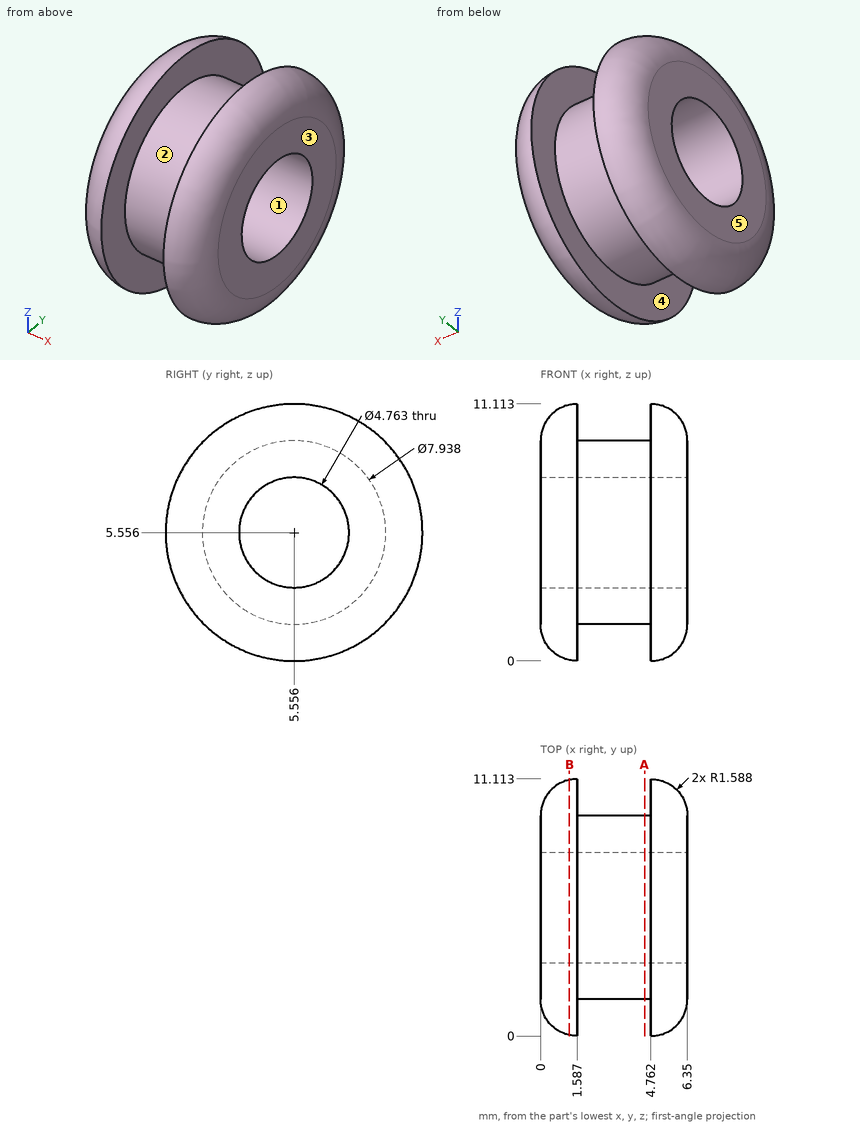
For this review, use the dimensioned drawing (mm, ordinates from the lowest corner) and the shaded views. A direction names the side the tool comes from. Give positions to 0.01 mm unless a question says otherwise; leave off trailing zeros. Order: outer loops, then holes, each group sorted by start corner. A loop starts at its lowest first (then second) coordinate and runs counter-clockwise, first axis right, second up. Notation, with made-up numbers: M 17.25,-3.5 L 60.25,-3.5 A27 ccw 60.25,32.5 Z; hole C -24.75,81 d1. An arc over 180 degrees is marked long. One line per question, with ' | ' between items. Start each with the question number.
1) Wall thickness on L1, parallel to Y at x = 3, z = 6 (1 decimal); L2, parallel to Z at x = 3.75, y = 6.75 (1 decimal): over which ranges is each line inside the solid? List them lowest first. Write a range as from..to.
2) Consider section B-B, the plane x = 1.25. Give the boundary of the cut face in (y, z).
3) For the marked faces 1 and 2, list the 3-axis set-ups (+Z, -Z, +X, -X, +Y, -Y) from which the entire face can be reached by the end or side of a thin tool; tool diameter is ignored.
4) Mouldability with a two-part tool opening along X and no side actions: class the marked faces 3, 4 and 5 as pulls with the +X half, pulls with the -X half, needs draft (parallel to the pull), parting line crosses it, or undercut.
5) Consider section A-A, the plane x = 4.5. Give the boundary of the cut face in (y, z) (1 decimal).
6) Clearance check with flat-ended pins moving along their axes: P1, Ø1.5, axis at x = 2.5, z = 2.5, coming from the +Y side (1 decimal); P2, Ø1.5, axis at x = 2.5, y = 3.5, coming from the +Z side; P3, Ø3, axis at x = 5.5, y = 8.5, coming from the -Z side. State where each tip first meets the part, or that it passes through.
Found:
1) L1: y = 1.6..3.2, 7.9..9.5 | L2: z = 1.8..3.5, 7.6..9.3
2) outline: C 5.56,5.56 d11.04; hole C 5.56,5.56 d4.76
3) face 1: +X, -X | face 2: none
4) face 3: pulls with the +X half | face 4: undercut | face 5: pulls with the -X half
5) outline: C 5.6,5.6 d7.9; hole C 5.6,5.6 d4.8
6) P1: stops at y = 8.8 | P2: stops at z = 9.3 | P3: stops at z = 0.23
